from build123d import *

# Parameters (mm, degrees)
SKETCH_1_R      = 60
SKETCH_1_R_2    = 3
EXTRUDE_1_DEPTH = 4


with BuildPart() as part:
    # 草图1 → 凸台-拉伸1 (new body)
    with BuildSketch(Plane.XY):
        Circle(SKETCH_1_R)
        Circle(SKETCH_1_R_2, mode=Mode.SUBTRACT)
        with BuildLine():
            Line((-4, 11.842719282), (-4, 50.341334905))
            ThreePointArc((-4, 50.341334905), (-43.734282891, 25.25), (-45.596874888, -21.706565837))
            Line((-45.596874888, -21.706565837), (-12.256095748, -2.457258026))
            ThreePointArc((-12.256095748, -2.457258026), (-10.825317547, 6.25), (-4, 11.842719282))
        make_face(mode=Mode.SUBTRACT)
        with BuildLine():
            Line((4, 11.842719282), (4, 50.341334905))
            ThreePointArc((4, 50.341334905), (43.734282891, 25.25), (45.596874888, -21.706565837))
            Line((45.596874888, -21.706565837), (12.256095748, -2.457258026))
            ThreePointArc((12.256095748, -2.457258026), (10.825317547, 6.25), (4, 11.842719282))
        make_face(mode=Mode.SUBTRACT)
        with BuildLine():
            Line((8.256095748, -9.385461256), (41.596874888, -28.634769068))
            ThreePointArc((41.596874888, -28.634769068), (0, -50.5), (-41.596874888, -28.634769068))
            Line((-41.596874888, -28.634769068), (-8.256095748, -9.385461256))
            ThreePointArc((-8.256095748, -9.385461256), (0, -12.5), (8.256095748, -9.385461256))
        make_face(mode=Mode.SUBTRACT)
    extrude(amount=EXTRUDE_1_DEPTH)


solid = part.part
Verification items for the finished model (mm, model axes). A direction names the side the tool comes from. Give positions to 0.01 mm unless a question says otherwise; leave off trailing zeros. Order: outer loops, then holes, each group sorted by start corner. A loop starts at its lowest first (then second) coordinate and runs counter-clockwise, first axis right, second up. Notation, with made-up numbers: M 38.5,40 L 96.5,40 A24 cw 96.5,73 Z; hole C -40,6 d9. An arc over 180 degrees is marked long. Use one line per item in the form item = value. Start each with the question number.
Q1. Section check A-A (y = 0). Enter the section's corners in (x, z), then the cut area to 3 significant figures.
Q2. Go/stop test with flat-tipped pins: pin 1 Ø1 at (x, z) = (-22.5, 2.5) entering from +Y; pin 2 Ø5 at (x, y) = (-19.5, -41.5) entering from -Z; pin 3 Ø2 at (y, z) = (28, 3) entering from +X; pin 4 Ø1.2 at (y, z) = (32.5, 2) entering from -X. Record where each tip stops, or that it passes through.
Q3. Access from +Z, -Z, +X, -X, +Y, -Y to the whole of each face (thin tool, end or side, straight path). Record for faces 1 (the flat face through (-5, 0, 0)), 2 (the cylindrical face through (43.39, 25.84, 1.97)).
Q4. Section check D-D (y = 21). Enter the section's corners in (x, z).
Q5. Scan lines: line 1 along Y through (x, z) = (0, 1.6); line 2 along X through (y, z) = (15, 2.8); line 3 along Y through (x, z) = (-36.5, 2.4). Record each from-to range of solid material in increasing order. Write a range as [from, to].
Q6. Section check B-B (x = 0). Enter the section's corners in (y, z).
Q7. Mould release check, pull along X, two halves, no side actions. Record for faces 3 (the cylindrical face through (-59.94, 2.64, 1.97)), 4 (the flat face through (-5, 0, 4)), 5 (the flat face through (-29.16, -12.217, 1.972)): +X half, -X half, draft (parallel to the pull), parting line (faces both ways), or undercut.
Q8. Section check C-C (z = 1.2). Enter the section's corners in (x, y), then the cut area to 3 significant figures.
Evaluation:
q1.outline = M -60,0 L -50.5,0 L -50.5,4 L -60,4 Z; M -12.5,0 L -3,0 L -3,4 L -12.5,4 Z; M 3,0 L 12.5,0 L 12.5,4 L 3,4 Z; M 50.5,0 L 60,0 L 60,4 L 50.5,4 Z
q1.area = 152 mm2
q2.pin_1 = 55.82
q2.pin_2 = through
q2.pin_3 = 53.58
q2.pin_4 = -50.82
q3.face_1 = -Z, +X, -X, +Y, -Y
q3.face_2 = +Z, -Z
q4.outline = M -56.2,0 L -45.93,0 L -45.93,4 L -56.2,4 Z; M -4,0 L 4,0 L 4,4 L -4,4 Z; M 45.93,0 L 56.2,0 L 56.2,4 L 45.93,4 Z
q5.line_1 = [-60, -50.5], [-12.5, -3], [3, 60]
q5.line_2 = [-58.09, -48.22], [-4, 4], [48.22, 58.09]
q5.line_3 = [-47.62, -34.9], [-25.69, -16.45], [34.9, 47.62]
q6.outline = M -60,0 L -50.5,0 L -50.5,4 L -60,4 Z; M -12.5,0 L -3,0 L -3,4 L -12.5,4 Z; M 3,0 L 60,0 L 60,4 L 3,4 Z
q7.face_3 = parting line
q7.face_4 = draft
q7.face_5 = undercut
q8.outline = C 0,0 d120; hole M -45.6,-21.71 L -12.26,-2.46 A12.5 cw -4,11.84 L -4,50.34 A50.5 ccw Z; hole M -41.6,-28.63 A50.5 ccw 41.6,-28.63 L 8.26,-9.39 A12.5 cw -8.26,-9.39 Z; hole C 0,0 d6; hole M 4,11.84 A12.5 cw 12.26,-2.46 L 45.6,-21.71 A50.5 ccw 4,50.34 Z
q8.area = 4,680 mm2
